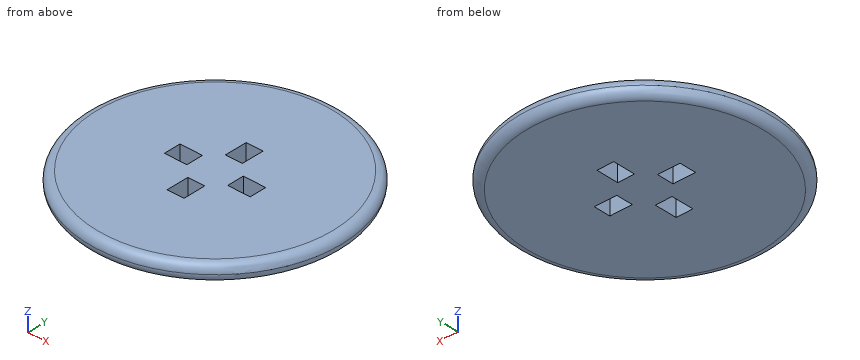
```python
from build123d import *

# Parameters (mm, degrees)
SKETCH1_R           = 45
SKETCH1_W           = 8
SKETCH1_H           = 6
SKETCH1_W_2         = 6
SKETCH1_H_2         = 8
BOSS_EXTRUDE1_DEPTH = 6
FILLET1_R           = 3
FILLET2_R           = 3


with BuildPart() as part:
    # Sketch1 → Boss-Extrude1 (new body)
    with BuildSketch(Plane.XY):
        Circle(SKETCH1_R)
        with Locations((11.25, 0)):
            Rectangle(SKETCH1_W, SKETCH1_H, mode=Mode.SUBTRACT)
        with Locations((0, -11.25)):
            Rectangle(SKETCH1_W_2, SKETCH1_H_2, mode=Mode.SUBTRACT)
        with Locations((-11.25, 0)):
            Rectangle(SKETCH1_W, SKETCH1_H, mode=Mode.SUBTRACT)
        with Locations((0, 11.25)):
            Rectangle(SKETCH1_W_2, SKETCH1_H_2, mode=Mode.SUBTRACT)
    extrude(amount=BOSS_EXTRUDE1_DEPTH)

    # Fillet1
    fillet1_edges = [part.edges().sort_by_distance(p)[0] for p in [
        (-45, 0, 6),
    ]]
    fillet(fillet1_edges, radius=FILLET1_R)

    # Fillet2
    fillet2_edges = [part.edges().sort_by_distance(p)[0] for p in [
        (-45, 0, 0),
    ]]
    fillet(fillet2_edges, radius=FILLET2_R - 0.0001)  # a hair under: the kernel refuses the full size


solid = part.part
```
CAD build for the part. Positions are in the model's coordinates, mm. Coordinates: 2 decimals unless noted, no trailing zeros. Write each loop counter-clockwise with the first axis right and the second up, starting at its lowest first coordinate (ties: lowest second). Pieces come first, ordered by that corner, then holes.
(1) Flat gauge pins, fed straight in: pin 1 (1.8 mm diameter, centred on x = -12.5, z = 2.5, fed in from +Y); pin 2 (1.5 mm diameter, centred on x = -29, y = -16, fed in from -Z); pin 3 (1.8 mm diameter, centred on x = 12, z = 3, fed in from +Y); pin 4 (3 mm diameter, centred on y = -10, z = 2, fed in from +X). Where does each tip first touch, or does it go through?
(2) Cut at C-C, the plane z = 1.5. List the corners of the cut face in (x, y).
(3) Drill centre lines: probe 1 along X at (y, z) = (9, 5); probe 2 along Y at (x, z) = (12, 4.05); probe 3 along X at (y, z) = (4, 1.7). Where is each one in solid material? Low to high.
(4) Cut at A-A, the plane y = 0. Count the separate pieces of the cut face and the enclosed holes in it, and give its area (3 significant figures).
Geometry says:
1. pin 1: stops at y = 43.46
1. pin 2: stops at z = 0
1. pin 3: stops at y = 43.61
1. pin 4: stops at x = 44.14
2. outline: circle Ø89.2 at (0, 0); hole (-15.25, -3) - (-7.25, -3) - (-7.25, 3) - (-15.25, 3) - close; hole (-3, -15.25) - (3, -15.25) - (3, -7.25) - (-3, -7.25) - close; hole (-3, 7.25) - (3, 7.25) - (3, 15.25) - (-3, 15.25) - close; hole (7.25, -3) - (15.25, -3) - (15.25, 3) - (7.25, 3) - close
3. probe 1: x = -43.31 to -3, 3 to 43.31
3. probe 2: y = -43.17 to -3, 3 to 43.17
3. probe 3: x = -44.52 to 44.52
4. separate pieces: 3
4. enclosed holes: 0
4. area: 436 mm2
